Solid Edge part; units mm, degrees
sketch "Sketch1" plane through (0, 0, 0) normal (0, 0, 1) x (1, 0, 0)
  line L0 (21.15, -21.15) -> (21.15, 21.15)
  line L1 (21.15, 21.15) -> (-21.15, 21.15)
  line L2 (-21.15, 21.15) -> (-21.15, -21.15)
  line L3 (-21.15, -21.15) -> (21.15, -21.15)
extrude "Protrusion1" add sketch "Sketch1" along normal blind 40
sketch "Sketch2" plane through (0, 0, 0) normal (0, 0, 1) x (1, 0, 0)
  circle A0 centre (0, 0) radius 11
extrude "ExtrudedProtrusion_2" add sketch "Sketch2" against normal blind 2
sketch "Sketch3" plane through (0, 0, 0) normal (0, 0, 1) x (1, 0, 0)
  circle A0 centre (0, 0) radius 4
extrude "ExtrudedProtrusion_3" add sketch "Sketch3" against normal blind 400
sketch "Sketch4" plane through (0, 0, 0) normal (0, 0, 1) x (1, 0, 0)
  circle A0 centre (15.5, 15.5) radius 1.5
  circle A1 centre (-15.5, 15.5) radius 1.5
  circle A2 centre (-15.5, -15.5) radius 1.5
  circle A3 centre (15.5, -15.5) radius 1.5
extrude "ExtrudedCutout_1" cut sketch "Sketch4" along normal blind 4.5
chamfer "Chamfer_1" distance 5 angle 45 4 edges at (21.15, 21.15, 20) (-21.15, 21.15, 20) (-21.15, -21.15, 20) (21.15, -21.15, 20)
fillet "Round_1" radius 1 8 edges at (0, 21.15, 40) (-18.65, 18.65, 40) (-21.15, 0, 40) (-18.65, -18.65, 40) (0, -21.15, 40) (18.65, -18.65, 40) (21.15, 0, 40) (18.65, 18.65, 40)
chamfer "Chamfer_2" distance 0.5 angle 45 1 edges at (-4, 0, -400)
Check sheet for the modelled part. Datum: model origin and axes. Units: mm. A direction names the side the tool comes from. Coordinates: 2 decimals unless noted, no trailing zeros. Order: outer loops, then holes, each group sorted by start corner. A loop starts at its lowest first (then second) coordinate and runs counter-clockwise, first axis right, second up. Notation, with made-up numbers: M 36,-38 L 41,-38 A16 cw 41,-34 Z; hole C 5.25,15 d8. An arc over 180 degrees is marked long. Write each question's results on one line, items separated by ' | '. Start each with the question number.
1. Go/stop test with flat-tipped pins: P1, Ø2.5, axis at x = -15.5, y = -15.5, coming from the -Z side; P2, Ø1.5, axis at x = -13.5, y = -1, coming from the -Z side; P3, Ø8, axis at x = 1.5, z = -355, coming from the +Y side. Record where each tip stops, or that it passes through.
2. Cross-section at A-A on z = -224.5. Record the cut outline in (x, y), and give its area (3 significant figures).
3. Material ranges on probe 1 along Y at (x, z) = (-15, 3); probe 2 along Y at (x, z) = (15.5, 2.5), recorded low to high.
4. Access from +Z, -Z, +X, -X, +Y, -Y to the whole of each face (thin tool, end or side, straight path). Record for faces 1 (the face through (21.15, 0, 19)), 2 (the face through (9, -9, 0)).
Checks:
1) P1: stops at z = 4.5 | P2: stops at z = 0 | P3: stops at y = 4
2) outline: C 0,0 d8 | area: 50.3 mm²
3) probe 1: y = -21.15 to -16.91, -14.09 to 14.09, 16.91 to 21.15 | probe 2: y = -21.15 to -17, -14 to 14, 17 to 21.15
4) face 1: +Z, -Z, +X, +Y, -Y | face 2: -Z
